Drawing for the job (mm, zero at the part's lowest x, y, z). A direction names the side the tool comes from. Give positions to 0.01 mm unless a question says otherwise; leave off trailing zeros. Order: outer loops, then holes, each group sorted by start corner. A loop starts at its lowest first (then second) coordinate and runs counter-clockwise, first axis right, second up. Notation, with made-up numbers: (28, -16) - (61, -16) arc R25 cw to (61, 8) - close; hole circle Ø6 at (74, -8). An arc over 180 degrees is marked (long way). Use a Markdown table: item, result. Add a question column.
(1) Slice it at C-C (y = 25). Write the cut outline in (x, z).
(2) Wall check: line 1 (Y direction, x = 115, z = 37); line 2 (Y direction, x = 115, z = 72.35); line 3 (X direction, y = 80.5, z = 49). Give the ranges that are in metal, low to high.
(3) Flat gauge pins, fed straight in: pin 1 (8 mm diameter, centred on x = 90.5, y = 87.5, fed in from +Z); pin 2 (6 mm diameter, centred on y = 22.5, z = 16.5, fed in from +X); pin 3 (1 mm diameter, centred on x = 194, z = 30, fed in from -Y). Where does each tip first touch, or does it go through?
(4) Slice it at B-B (x = 115). Write the cut outline in (y, z), then the cut area to 4 significant figures.
(5) Which spindle directions (+Z, -Z, +X, -X, +Y, -Y) get a long thin tool onto all of the face, cutting with end or side? Do the marked faces 5, 6 and 7. Say none if no direction does.
(6) Mould opens along X. For the marked faces 1, 2, 3 and 4 say: +X half, -X half, draft (parallel to the pull), parting line (faces both ways), or undercut.
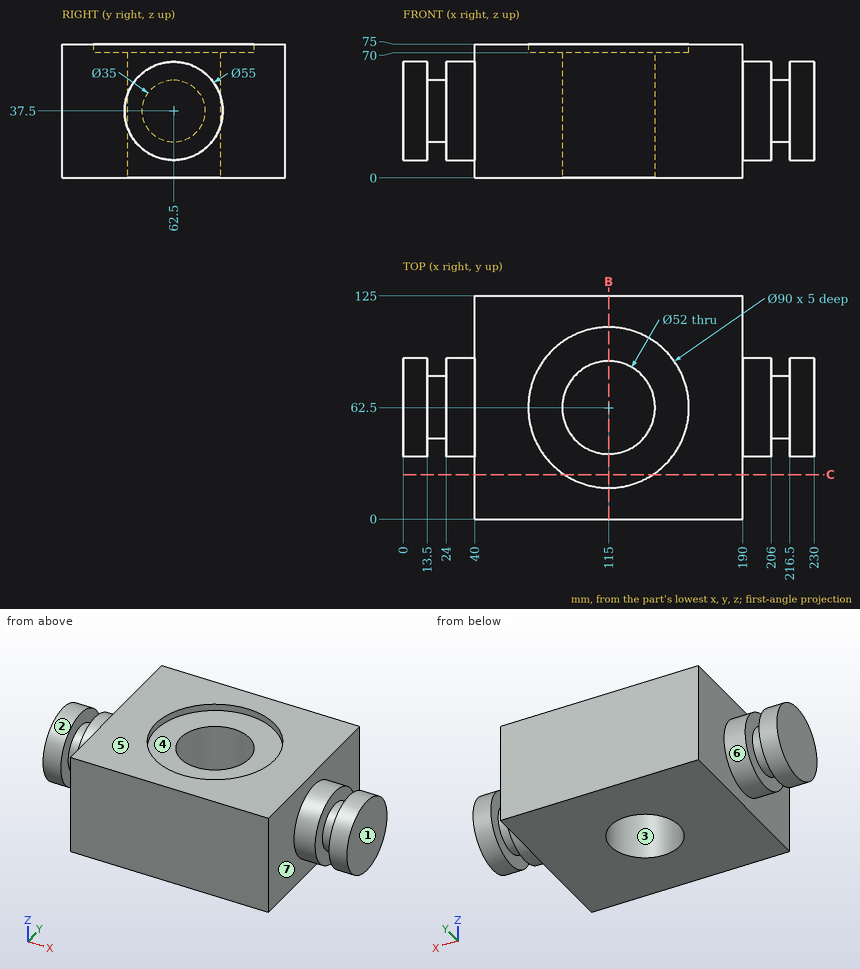
Solution:
| question | item | result |
|---|---|---|
| 1 | outline | (40, 0) - (190, 0) - (190, 75) - (139.87, 75) - (139.87, 70) - (90.13, 70) - (90.13, 75) - (40, 75) - close |
| 2 | line 1 | 0 to 36.5, 88.5 to 125 |
| 2 | line 2 | 0 to 17.5, 107.5 to 125 |
| 2 | line 3 | 0 to 13.5, 24 to 96.24, 133.76 to 206, 216.5 to 230 |
| 3 | pin 1 | z = 70 |
| 3 | pin 2 | x = 190 |
| 3 | pin 3 | y = 35.91 |
| 4 | outline | (0, 0) - (36.5, 0) - (36.5, 70) - (17.5, 70) - (17.5, 75) - (0, 75) - close; (88.5, 0) - (125, 0) - (125, 75) - (107.5, 75) - (107.5, 70) - (88.5, 70) - close |
| 4 | area | 5,285 mm2 |
| 5 | face 5 | +Z, +X, -X, +Y, -Y |
| 5 | face 6 | -X |
| 5 | face 7 | +X |
| 6 | face 1 | +X half |
| 6 | face 2 | draft |
| 6 | face 3 | undercut |
| 6 | face 4 | undercut |
